Model file for the job. Use its own axes, mm. A direction names the side the tool comes from. Give positions to 0.01 mm unless a question says otherwise; leave off trailing zeros. Loops run counter-clockwise (first coordinate to the right, second up) from the corner with the lowest first, then second, coordinate; pieces in that order, holes last. Notation, with made-up numbers: M 1,22.25 L 33,22.25 A25 cw 33,43.25 Z; hole C 20,48 d2. An arc over 180 degrees is marked long. Answer in a Markdown table with one row per item.
```python
from build123d import *

# Parameters (mm, degrees)
SKETCH_1_R               = 15
EXTRUDE_1_DEPTH          = 2000
EXTRUDE_1_2_DEPTH        = 2000
SKETCH_2_R               = 15
EXTRUDE_2_DEPTH          = 2000
CUT_EXTRUDE_1_DEPTH      = 2018.973628535
CUT_EXTRUDE_1_DEPTH_BACK = 2018.973628535
SKETCH_3_R               = 3
SKETCH_6_W               = 535.348800536
SKETCH_6_H               = 30
EXTRUDE_3_DEPTH          = 3


with BuildPart() as part:
    # Sketch 1 → Extrude 1 (new body)
    with BuildSketch(Plane.XY):
        with Locations((-250, 0)):
            Circle(SKETCH_1_R)
    extrude(amount=EXTRUDE_1_DEPTH)



with BuildPart() as body_2:
    # Sketch 1 → Extrude 1 2 (new body)
    with BuildSketch(Plane.XY):
        with Locations((250, 0)):
            Circle(SKETCH_1_R)
    extrude(amount=EXTRUDE_1_2_DEPTH)


with BuildPart() as part_1:
    add(part.part)

    add(body_2.part)  # Extrude 2 merges body 2
    # Sketch 2 → Extrude 2 (add)
    with BuildSketch(Plane(origin=(0, 0, 0), x_dir=(-1, 0, 0), z_dir=(0, 0, -1))):
        with BuildLine():
            Line((-232.09413573, 1.83848436), (232.09413573, 1.83848436))
            ThreePointArc((232.09413573, 1.83848436), (267.996794905, -0.339666233), (232.037514609, -1.16151564))
            Line((232.037514609, -1.16151564), (-232.037514609, -1.16151564))
            ThreePointArc((-232.037514609, -1.16151564), (-267.996794905, -0.339666233), (-232.09413573, 1.83848436))
        make_face()
        with Locations((-250, 0)):
            Circle(SKETCH_2_R, mode=Mode.SUBTRACT)
        with Locations((250, 0)):
            Circle(SKETCH_2_R, mode=Mode.SUBTRACT)
    extrude(amount=-EXTRUDE_2_DEPTH)

    # Sketch 3 → Cut-Extrude 1 (cut, two sides: drawn at the far end of the back side and taken through both)
    with BuildSketch(Plane(origin=(0, 1.83848436, 0), x_dir=(1, 0, 0), z_dir=(0, 1, 0)).offset(-CUT_EXTRUDE_1_DEPTH_BACK)):
        with Locations(Location((250.018757305, -150, 0), (0, 0, 180))):
            Circle(SKETCH_3_R)
        with Locations(Location((-250.018757305, -150, 0), (0, 0, 180))):
            Circle(SKETCH_3_R)
    extrude(amount=CUT_EXTRUDE_1_DEPTH + CUT_EXTRUDE_1_DEPTH_BACK, mode=Mode.SUBTRACT)

    # Sketch 6 → Extrude 3 (add)
    with BuildSketch(Plane(origin=(0, 18, 0), x_dir=(1, 0, 0), z_dir=(0, 1, 0))):
        with Locations((-0.325599732, -308.023795678)):
            Rectangle(SKETCH_6_W, SKETCH_6_H)
        with Locations((-0.325599732, -1668.181126051)):
            Rectangle(SKETCH_6_W, SKETCH_6_H)
    extrude(amount=-EXTRUDE_3_DEPTH)


solid = part_1.part
```
Q1. Probe probe 1 along X at (y, z) = (-1, 150); probe 2 along X at (y, z) = (11, 150); probe 3 along X at (y, z) = (5, 150). List the from-to ranges inside material, lowest first.
Reported:
| item | result |
|---|---|
| probe 1 | -267.97 to -253.02, -247.02 to 247.02, 253.02 to 267.97 |
| probe 2 | -264.25 to -253.02, -247.02 to -235.75, 235.75 to 247.02, 253.02 to 264.25 |
| probe 3 | -267.29 to -253.02, -247.02 to -232.71, 232.71 to 247.02, 253.02 to 267.29 |
Q2. Mould opens along X. For faces 3 (the face through (-1, 0, 0)), 4 (the face through (-3, -1.162, 986)) say: released by +X, released by -X, zero draft, split by the parting line, or undercut.
Reported:
| item | result |
|---|---|
| face 3 | zero draft |
| face 4 | undercut |
Q3. Drop flat-ended pins along their axis: pin 1 (2 mm diameter, centred on x = 264, z = 1671, fed in from -Y); pin 2 (12 mm diameter, centred on x = 164.5, y = 2, fed in from -Z); pin 3 (5 mm diameter, centred on x = -205.5, z = 957.5, fed in from +Y); pin 4 (1.5 mm diameter, centred on y = -1, z = 1122.5, fed in from -X). Give the stop position or say it passes through.
Reported:
| item | result |
|---|---|
| pin 1 | y = -12.45 |
| pin 2 | z = 0 |
| pin 3 | y = 1.84 |
| pin 4 | x = -268 |
Q4. 3-axis set-ups, long thin cutter, end or side, ignore diameter. For faces 1 (the face through (263.28, -12.15, 986)), 2 (the face through (-1, 0, 2000)): which of +Z, -Z, +X, -X, +Y, -Y reach the whole face in a straight line?
Reported:
| item | result |
|---|---|
| face 1 | none |
| face 2 | +Z, +X, -X, +Y, -Y |
Q5. Saw through at B-B (y = -7). Give the cut face in (x, z), and give its area (3 significant figures).
Reported:
| item | result |
|---|---|
| outline | M -266.58,0 L -233.42,0 L -233.42,2000 L -266.58,2000 Z; M 233.42,0 L 266.58,0 L 266.58,2000 L 233.42,2000 Z; hole C -250.02,150 d6; hole C 250.02,150 d6 |
| area | 133,000 mm² |
Q6. Saw through at A-A (x = 35). Give the cut face in (y, z).
Reported:
| item | result |
|---|---|
| outline | M -1.16,0 L 1.84,0 L 1.84,2000 L -1.16,2000 Z; M 15,293.02 L 18,293.02 L 18,323.02 L 15,323.02 Z; M 15,1653.18 L 18,1653.18 L 18,1683.18 L 15,1683.18 Z |
